Geometry check sheet. Reference: the model listing, model coordinates, mm. Give positions to 0.01 mm unless a question says otherwise; leave off trailing zeros. Write each loop counter-clockwise with the first axis right and the second up, starting at its lowest first coordinate (ties: lowest second). Pieces come first, ordered by that corner, then holes.
(1) Cross-section at A-A (y = 17). Record the boundary of the cut face in (x, z), and give its area (3 significant figures).
(2) Depth check by flat-ended pin: P1, Ø1.5, axis at y = 51, z = -3.5, coming from the -X side; P2, Ø1, axis at x = -1, z = -3.5, coming from the -Y side; P3, Ø4, axis at y = 7, z = -4, coming from the -X side; P4, Ø2, axis at y = 39.5, z = 1.5, coming from the +X side. Enter the tip coordinate at first touch or a pass-through.
(3) Thickness scan on line 1 along Z through (x, y) = (4, 19); line 2 along Z through (x, y) = (1.75, 30); line 3 along X through (y, z) = (45, -0.25). Record the ranges inside material, lowest first.
Autodesk Inventor part; units mm, degrees
ref_plane "YZ Plane" through (0, 0, 0) normal (1, 0, 0) x (0, 1, 0)
ref_plane "XZ Plane" through (0, 0, 0) normal (0, 1, 0) x (-1, 0, 0)
ref_plane "XY Plane" through (0, 0, 0) normal (0, 0, 1) x (1, 0, 0)
sketch "Boceto1" plane through (0, 0, 0) normal (0, 1, 0) x (-1, 0, 0)
  circle A0 centre (0.3797, 0) radius 5
  point P0 (0, 0)
  dimension "d0" = 10
extrude "Extrusión1" add sketch "Boceto1" along normal blind 60
chamfer "Chaflán1" distance 0.5 angle 45 1 edges at (4.6203, 60, 0)
chamfer "Chaflán2" distance 0.5 angle 45 1 edges at (4.6203, 0, 0)
properties part number "EJE"
Reply:
1. outline: circle Ø10 at (-0.38, 0)
1. area: 78.5 mm2
2. P1: stops at x = -4.56
2. P2: stops at y = 0
2. P3: stops at x = -4.96
2. P4: stops at x = 4.6
3. line 1: z = -2.41 to 2.41
3. line 2: z = -4.52 to 4.52
3. line 3: x = -5.37 to 4.61
